Study the drawing (mm; zero at the part's minimum x, y, z) and answer. Round coordinates to 2 decimals unless told otherwise and drop trailing zeros. Write each loop counter-clockwise with the first axis right and the second up, starting at its lowest first coordinate (ties: lowest second). Pieces come first, ordered by that corner, then holes. Notation, with made-up numbers: (68.5, 59) - (83.5, 59) arc R14 cw to (83.5, 80) - close; hole circle Ø1 at (26.5, 70). An arc over 180 degrees is marked (long way). Return JSON: item names as keys, results as strings. Group by question number.
(1) Find the intervals of material crossed by line 1 along X through (y, z) = (2, 1.5); line 2 along Y through (x, z) = (2, 1.05); line 3 along X through (y, z) = (41, 1.7), in increasing order. Write a range as [from, to].
(2) Each of these flat-tipped pins is pushed along its axis until it touches: pin 1 (1.5 mm diameter, centred on x = 15.5, z = 1, fed in from +Y); pin 2 (0.9 mm diameter, centred on y = 5.5, z = 1.5, fed in from +X); pin 3 (1.5 mm diameter, centred on y = 6.5, z = 1.5, fed in from -X). Where does it stop, or does it pass through?
(3) Section A-A, the plane x = 14 is taken. Write down the section's boundary in (y, z).
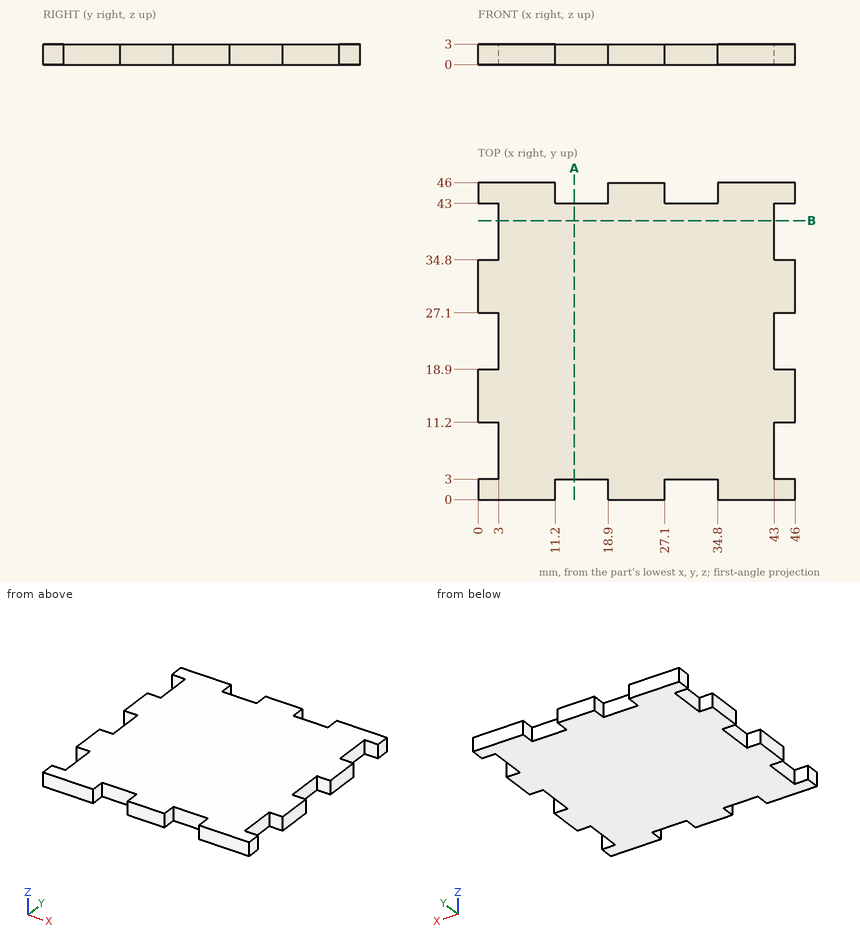
Working result:
{
 "1": {"line 1": "x = [0, 11.2], [18.9, 27.1], [34.8, 46]", "line 2": "y = [0, 3], [11.2, 18.9], [27.1, 34.8], [43, 46]", "line 3": "x = [3, 43]"},
 "2": {"pin 1": "stops at y = 43", "pin 2": "stops at x = 43", "pin 3": "stops at x = 3"},
 "3": {"outline": "(3, 0) - (43, 0) - (43, 3) - (3, 3) - close"}
}
